Verification items for the finished model (mm, model axes). Face numbers are marked on the shaded views. A direction names the side the tool comes from. Coordinates: 2 decimals unless noted, no trailing zeros. Write each loop counter-clockwise with the first axis right and the second up, starting at its lowest first coordinate (ties: lowest second). Pieces come first, ordered by that corner, then holes. Notation, with made-up numbers: M -24,-3.5 L -4,-3.5 A21 ccw -4,1.5 Z; hole C -32.75,-17.5 d10. An arc over 180 degrees is marked long. Answer in a Markdown table with one row per item.
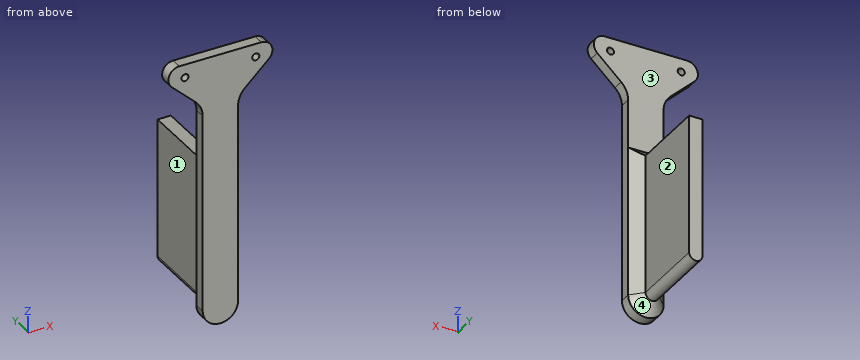
from build123d import *

# Parameters (mm, degrees)
SKETCH1_R           = 1
BOSS_EXTRUDE1_DEPTH = 3
BOSS_EXTRUDE2_DEPTH = 40
CHAMFER1_SIZE       = 5
SKETCH3_R           = 1.6
CUT_EXTRUDE1_DEPTH  = 10
BOSS_EXTRUDE3_START = -3
SKETCH4_R           = 1
BOSS_EXTRUDE3_DEPTH = 3
BOSS_EXTRUDE4_START = 2
SKETCH5_R           = 1.6
BOSS_EXTRUDE4_DEPTH = 2


with BuildPart() as part:
    # Sketch1 → Boss-Extrude1 (new body)
    with BuildSketch(Plane(origin=(0, 0, 0), x_dir=(1, 0, 0), z_dir=(0, 1, 0))):
        with BuildLine():
            Line((-18.528780813, -6), (18.528780813, -6))
            ThreePointArc((18.528780813, -6), (23.17842758, -2.838691096), (21.948486458, 2.647686021))
            Line((21.948486458, 2.647686021), (11.160588711, 12.761340158))
            ThreePointArc((11.160588711, 12.761340158), (8.824104597, 16.081420568), (8, 20.056712199))
            Line((8, 20.056712199), (8, 95))
            Line((8, 95), (8, 110))
            ThreePointArc((8, 110), (0, 118), (-8, 110))
            Line((-8, 110), (-8, 95))
            Line((-8, 95), (-8, 20.056712199))
            ThreePointArc((-8, 20.056712199), (-8.824104597, 16.081420568), (-11.160588711, 12.761340158))
            Line((-11.160588711, 12.761340158), (-21.948486458, 2.647686021))
            ThreePointArc((-21.948486458, 2.647686021), (-23.17842758, -2.838691096), (-18.528780813, -6))
        make_face()
        with Locations(Location((0, 15, 0), (0, 0, 270))):
            Circle(SKETCH1_R, mode=Mode.SUBTRACT)
        with Locations(Location((-16, 0, 0), (0, 0, 270))):
            Circle(SKETCH1_R, mode=Mode.SUBTRACT)
        with Locations(Location((16, 0, 0), (0, 0, 270))):
            Circle(SKETCH1_R, mode=Mode.SUBTRACT)
    extrude(amount=BOSS_EXTRUDE1_DEPTH)

    # Sketch2 → Boss-Extrude2 (add)
    with BuildSketch(Plane(origin=(0, 3, 0), x_dir=(1, 0, 0), z_dir=(0, 1, 0))):
        with BuildLine():
            Line((3, 47), (-3, 47))
            Line((-3, 47), (-3, 95))
            Line((-3, 95), (-3, 110))
            ThreePointArc((-3, 110), (0, 113), (3, 110))
            Line((3, 110), (3, 95))
            Line((3, 95), (3, 47))
        make_face()
    extrude(amount=BOSS_EXTRUDE2_DEPTH)

    # Chamfer1
    chamfer1_edges = [part.edges().sort_by_distance(p)[0] for p in [
        (3, 3, -78.5),
        (0, 3, -113),
        (-3, 3, -78.5),
        (0, 3, -47),
    ]]
    chamfer(chamfer1_edges, length=CHAMFER1_SIZE - 0.0001)  # a hair under: the kernel refuses the full size

    # Sketch3 → Cut-Extrude1 (cut)
    with BuildSketch(Plane(origin=(0, 3, 0), x_dir=(1, 0, 0), z_dir=(0, 1, 0))):
        with Locations(Location((-16, 0, 0), (0, 0, 270))):
            Circle(SKETCH3_R)
        with Locations(Location((16, 0, 0), (0, 0, 270))):
            Circle(SKETCH3_R)
    extrude(amount=-CUT_EXTRUDE1_DEPTH, mode=Mode.SUBTRACT)

    # Sketch4 → Boss-Extrude3 (add)
    with BuildSketch(Plane(origin=(0, 3, 0), x_dir=(1, 0, 0), z_dir=(0, 1, 0)).offset(BOSS_EXTRUDE3_START)):
        with Locations((0, 15)):
            Circle(SKETCH4_R)
    extrude(amount=BOSS_EXTRUDE3_DEPTH)

    # Sketch5 → Boss-Extrude4 (add)
    with BuildSketch(Plane.XZ.offset(BOSS_EXTRUDE4_START)):
        with BuildLine():
            Line((11.160588711, -12.761340158), (21.948486458, -2.647686021))
            ThreePointArc((21.948486458, -2.647686021), (23.17842758, 2.838691096), (18.528780813, 6))
            Line((18.528780813, 6), (-18.528780813, 6))
            ThreePointArc((-18.528780813, 6), (-23.17842758, 2.838691096), (-21.948486458, -2.647686021))
            Line((-21.948486458, -2.647686021), (-11.160588711, -12.761340158))
            ThreePointArc((-11.160588711, -12.761340158), (-8.824104597, -16.081420568), (-8, -20.056712199))
            Line((-8, -20.056712199), (-8, -110))
            ThreePointArc((-8, -110), (0, -118), (8, -110))
            Line((8, -110), (8, -20.056712199))
            ThreePointArc((8, -20.056712199), (8.824104597, -16.081420568), (11.160588711, -12.761340158))
        make_face()
        with Locations(Location((-16, 0, 0), (0, 0, 90))):
            Circle(SKETCH5_R, mode=Mode.SUBTRACT)
        with Locations(Location((16, 0, 0), (0, 0, 90))):
            Circle(SKETCH5_R, mode=Mode.SUBTRACT)
    extrude(amount=-BOSS_EXTRUDE4_DEPTH)


solid = part.part
1) Tool access check on the marked faces 1, 2, 3 and 4. Record the directions out of +Z, -Z, +X, -X, +Y, -Y that give a thin tool (end or side, any length) a straight path to the whole face; none if there is none.
Response values:
| item | result |
|---|---|
| face 1 | +Z, -Z, -X, +Y |
| face 2 | +Z, -Z, +X, +Y |
| face 3 | +Z, +X, -X, +Y |
| face 4 | -Z, +Y |
2) Thickness scan on L1, parallel to X at y = 0, z = 0; L2, parallel to X at y = 9, z = -52.5; L3, parallel to X at y = 1.5, z = -79. Record the ranges inside material, lowest first. Write a range as [from, to].
Response values:
| item | result |
|---|---|
| L1 | x = [-23.43, -17.6], [-14.4, 14.4], [17.6, 23.43] |
| L2 | x = [-3, 3] |
| L3 | x = [-8, 8] |
3) Sectioned sample at A-A (z = 0). Record the cut outline in (x, y).
Response values:
| item | result |
|---|---|
| outline | M -23.43,-2 L -17.6,-2 L -17.6,3 L -23.43,3 Z; M -14.4,-2 L 14.4,-2 L 14.4,3 L -14.4,3 Z; M 17.6,-2 L 23.43,-2 L 23.43,3 L 17.6,3 Z |
4) Depth check by flat-ended pin: pin 1 (2.5 mm diameter, centred on y = 0, z = -65, fed in from -X); pin 2 (2.5 mm diameter, centred on y = 0, z = -46, fed in from +X); pin 3 (23.5 mm diameter, centred on x = -11, z = -83.5, fed in from +Y); pin 4 (10.5 mm diameter, centred on y = 34, z = -75.5, fed in from -X). Enter the tip coordinate at first touch or a pass-through.
Response values:
| item | result |
|---|---|
| pin 1 | stops at x = -8 |
| pin 2 | stops at x = 8 |
| pin 3 | stops at y = 43 |
| pin 4 | stops at x = -3 |
5) Sectioned sample at B-B (x = 16). Record the cut outline in (y, z).
Response values:
| item | result |
|---|---|
| outline | M -2,-8.22 L 3,-8.22 L 3,-1.6 L -2,-1.6 Z; M -2,1.6 L 3,1.6 L 3,6 L -2,6 Z |
